from build123d import *

# Parameters (mm, degrees)
EXTRUDE_1_DEPTH = 4
SKETCH_2_R      = 3
EXTRUDE_2_DEPTH = 20
CHAMFER_2_SIZE  = 1


with BuildPart() as part:
    # Эскиз1 → Вытянуть1 (new body)
    with BuildSketch(Plane(origin=(0, 0, 0), x_dir=(1, 0, 0), z_dir=(0, 1, 0))):
        Polygon((-2.886751346, 5), (2.886751346, 5), (5.773502692, 0), (2.886751346, -5), (-2.886751346, -5), (-5.773502692, 0), align=None)
    extrude(amount=-EXTRUDE_1_DEPTH)

    # Эскиз2 → Вытянуть2 (add)
    with BuildSketch(Plane.XZ.offset(4)):
        with Locations(Location((0, 0, 0), (0, 0, 270))):
            Circle(SKETCH_2_R)
    extrude(amount=EXTRUDE_2_DEPTH)

    # Фаска2
    chamfer_2_edges = [part.edges().sort_by_distance(p)[0] for p in [
        (0, -24, 3),
    ]]
    chamfer(chamfer_2_edges, length=CHAMFER_2_SIZE)

    # Эскиз3 → Вырез-Повернуть1 (revolve, cut)
    with BuildSketch(Plane.XY, mode=Mode.PRIVATE) as cut_revolve_1_sk:
        Polygon((-5.773502692, -1), (-4.773502692, 0), (-5.773502692, 0), align=None)
        Polygon((-5.773502692, -3), (-4.773502692, -4), (-5.773502692, -4), align=None)
    revolve(cut_revolve_1_sk.sketch.rotate(Axis((0, -4, 0), (0, -1, 0)), 270), axis=Axis((0, -4, 0), (0, -1, 0)), mode=Mode.SUBTRACT)


solid = part.part
Build history of the part. All positions in model axes, mm. A direction names the side the tool comes from. Give positions to 0.01 mm unless a question says otherwise; leave off trailing zeros. Loops run counter-clockwise (first coordinate to the right, second up) from the corner with the lowest first, then second, coordinate; pieces in that order, holes last. Notation, with made-up numbers: (65.5, 48.25) - (82.5, 48.25) arc R4 ccw to (82.5, 55.25) - close; hole circle Ø10 at (41, 28.5). An arc over 180 degrees is marked (long way). Write item = value, one per line. Start each with the question number.
1) Probe probe 1 along Y at (x, z) = (-3.5, -3); probe 2 along X at (y, z) = (-9.5, -0.5); probe 3 along Y at (x, z) = (-2.5, 4.5). List the from-to ranges inside material, lowest first. Write a range as from..to.
2) Drop flat-ended pins along their axis: pin 1 Ø1 at (y, z) = (-13, -1) entering from +X; pin 2 Ø6 at (x, z) = (-4, 1) entering from -Y; pin 3 Ø3 at (y, z) = (-14, -3.5) entering from +X. Give the stop position or say it passes through.
3) Band-saw the part on B-B on y = -1.5. Give the cut face in (x, z).
4) Band-saw the part on A-A on x = 0. Give the cut face in (y, z).
5) Tool access for faces 4 (the flat face through (-1, -4, 3)), 5 (the flat face through (0, -2, -5)): list every direction of +Z, -Z, +X, -X, +Y, -Y with a clear straight run to the whole face (end or side of a thin tool).
6) Pull direction Y, two halves, no side cores. Call faces 1 (the flat face through (-4.31, -1.975, 2.535)), 2 (the flat face through (0, -24, 0)), 3 (the flat face through (0, 0, 0)): +Y half, -Y half, draft (parallel to the pull), parting line (faces both ways), or undercut.
7) Band-saw the part on C-C on y = -6. Give the cut face in (x, z).
Final values:
q1.probe_1 = -4..0
q1.probe_2 = -2.96..2.96
q1.probe_3 = -3.63..-0.37
q2.pin_1 = 2.96
q2.pin_2 = -24
q2.pin_3 = 2.24
q3.outline = (-5.77, 0) - (-2.89, -5) - (2.89, -5) - (5.77, 0) - (2.89, 5) - (-2.89, 5) - close
q4.outline = (-24, -2) - (-23, -3) - (-4, -3) - (-4, -4.77) - (-3.77, -5) - (-0.23, -5) - (0, -4.77) - (0, 4.77) - (-0.23, 5) - (-3.77, 5) - (-4, 4.77) - (-4, 3) - (-23, 3) - (-24, 2) - close
q5.face_4 = -Y
q5.face_5 = -Z, +X, -X, +Y, -Y
q6.face_1 = draft
q6.face_2 = -Y half
q6.face_3 = +Y half
q7.outline = circle Ø6 at (0, 0)
